Source: CAD feature listing. Evaluate the final solid. Frame: model axes, mm. Coordinates: 2 decimals unless noted, no trailing zeros. Order: outer loops, then holes, each group sorted by start corner. A loop starts at its lowest first (then second) coordinate and runs counter-clockwise, first axis right, second up. Notation, with made-up numbers: (-35, -2.5) -> (3, -2.5) arc R18 cw to (3, 24.5) -> close; hole circle Ø3 at (60, 21.25). An arc over 180 degrees is marked (long way). Write item = value, one per line. Start each with the question number.
Item 1: Ray query, line 1 along Z through (x, y) = (7, -11.5); line 2 along X through (y, z) = (-11.5, 383); line 3 along X through (y, z) = (-13.75, 1154). Return the intervals inside material, ascending. Write a range as [from, to].
Item 2: Contact query for a flat-ended pin moving along its axis: pin 1 (3 mm diameter, centred on x = 414, z = 401.5, fed in from +Y). Output: stop coordinate, or through.
Item 3: Section query B-B (x = -233). Output: boundary loops of the cut face in (y, z), then the cut area to 3 significant figures.
Item 4: Section query A-A (z = 692.5). Output: boundary loops of the cut face in (x, y).
```python
from build123d import *

# Parameters (mm, degrees)
F1_DEPTH = 18
F2_R     = 300
F4_DEPTH = 25
F5_R     = 200


with BuildPart() as f1:
    # F0 (on Front) → F1 (new body)
    with BuildSketch(Plane.XZ):
        with BuildLine():
            Line((-685, 200), (-685, 0))
            Line((-685, 0), (685, 0))
            Line((685, 0), (685, 200))
            ThreePointArc((685, 200), (673.746048, 800.421727), (640, 1400))
            ThreePointArc((640, 1400), (0, 1500), (-640, 1400))
            ThreePointArc((-640, 1400), (-673.746048, 800.421727), (-685, 200))
        make_face()
    extrude(amount=F1_DEPTH)

    # F2
    f2_edges = [f1.edges().sort_by_distance(p)[0] for p in [
        (-640, -9, 1400),
        (640, -9, 1400),
    ]]
    fillet(f2_edges, radius=F2_R)

    # F3 (on face) → F4 (cut)
    with BuildSketch(Plane.XZ.offset(18)):
        Polygon((400, 1250), (-400, 1250), (-375, 200), (375, 200), align=None)
    extrude(amount=-F4_DEPTH, mode=Mode.SUBTRACT)

    # F5
    f5_edges = [f1.edges().sort_by_distance(p)[0] for p in [
        (400, -9, 1250),
        (-400, -9, 1250),
        (-375, -9, 200),
        (375, -9, 200),
    ]]
    fillet(f5_edges, radius=F5_R)


solid = f1.part
```
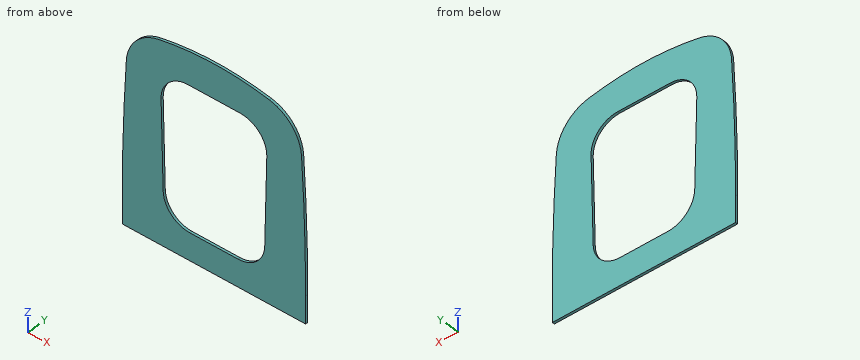
Computed:
q1.line_1 = [0, 200], [1250, 1499.99]
q1.line_2 = [-683.95, -378.98], [378.98, 683.95]
q1.line_3 = [-656.57, -366.01], [366.01, 656.57]
q2.pin_1 = 0
q3.outline = (-18, 0) -> (0, 0) -> (0, 207.23) -> (-18, 207.23) -> close; (-18, 1246.39) -> (0, 1246.39) -> (0, 1487.02) -> (-18, 1487.02) -> close
q3.area = 8,060 mm^2
q4.outline = (-677.43, -18) -> (-386.73, -18) -> (-386.73, 0) -> (-677.43, 0) -> close; (386.73, -18) -> (677.43, -18) -> (677.43, 0) -> (386.73, 0) -> close
